Autodesk Inventor part; units mm, degrees
ref_plane "YZ Plane" through (0, 0, 0) normal (1, 0, 0) x (0, 1, 0)
ref_plane "XZ Plane" through (0, 0, 0) normal (0, 1, 0) x (-1, 0, 0)
ref_plane "XY Plane" through (0, 0, 0) normal (0, 0, 1) x (1, 0, 0)
sketch "Boceto1" plane through (0, 0, 0) normal (0, 1, 0) x (-1, 0, 0)
  circle A0 centre (0, 0) radius 34.5
  circle A1 centre (0, 0) radius 35
  dimension "d0" = 69
  dimension "d1" = 70
extrude "Extrusión1" add sketch "Boceto1" along normal blind 1 contours A0 | A1
sketch "Boceto2" plane through (0, 1, 0) normal (0, 1, 0) x (1, 0, 0)
  circle A0 centre (0, 0) radius 34.5
  circle A1 centre (0, 0) radius 35
  dimension "d4" = 69
  dimension "d5" = 70
extrude "Extrusión2" add sketch "Boceto2" along normal blind 25
sketch "Boceto3" plane through (0, 1, 0) normal (0, 1, 0) x (1, 0, 0)
  circle A0 centre (0, 0) radius 2.1
  circle A1 centre (0, 0) radius 1.75
  dimension "d8" = 4.2
  dimension "d9" = 3.5
extrude "Extrusión3" add sketch "Boceto3" along normal blind 3
sketch "Boceto4" plane through (0, 1, 0) normal (0, 1, 0) x (1, 0, 0)
  circle A0 centre (0, 0) radius 1.75
  dimension "d14" = 3.5
extrude "Extrusión4" cut sketch "Boceto4" against normal through all
properties part number "Molde"
Could you check a few things on this model? Use its own coordinates, in mm. A direction names the side the tool comes from. Coordinates: 2 decimals unless noted, no trailing zeros. Order: outer loops, then holes, each group sorted by start corner. A loop starts at its lowest first (then second) coordinate and runs counter-clockwise, first axis right, second up. Notation, with made-up numbers: M 41,-3.5 L 76,-3.5 A5 ccw 76,1.5 Z; hole C 89.25,42 d8. An arc over 180 degrees is marked long. Use a Markdown table: item, result. Add a question column.
Q1. I want a section at A-A on z = 0. List the corners of the cut face in (x, y) for me, then the cut area to 3 significant figures.
Q2. We'd pull the mould along Z, two halves only. Please class faces 1 (the cylindrical face through (32.907, 13.325, 10.363)), 2 (the flat face through (26, 26, 23)): pulls with the +Z half, pulls with the -Z half, needs draft (parallel to the pull), parting line crosses it, or undercut.
Q3. If I drill on L1, parallel to Z at x = 0, y = 2.95; L2, parallel to X at y = 0.6, z = 0; L3, parallel to Z at x = 0, y = 15.25, over which ranges is the centre line in solid material (lowest first)?
Q4. I'm going to push flat-ended pins straight in: pin 1 (5 mm diameter, centred on y = 4, z = -25.5, fed in from +X); pin 2 (1 mm diameter, centred on y = 3.5, z = -19.5, fed in from -X); pin 3 (5 mm diameter, centred on x = 24, y = 7, fed in from +Z). Where does each tip first touch, or does it pass through?
Q5. Which directions (+Z, -Z, +X, -X, +Y, -Y) give clear straight access to the entire face, cutting with the end or side of a thin tool? Please do faces 3 (the flat face through (0, 1, -7)), 4 (the flat face through (0, 0, -7)).
Q6. I want a section at D-D on y = 17. List the corners of the cut face in (x, z) for me.
Q7. I want a section at C-C on y = 2.5. List the corners of the cut face in (x, z) for me, then the cut area to 3 significant figures.
Q8. I want a section at B-B on x = 0. List the corners of the cut face in (y, z) for me.
Checked values:
| question | item | result |
|---|---|---|
| 1 | outline | M -35,0 L -1.75,0 L -1.75,4 L -2.1,4 L -2.1,1 L -34.5,1 L -34.5,26 L -35,26 Z; M 1.75,0 L 35,0 L 35,26 L 34.5,26 L 34.5,1 L 2.1,1 L 2.1,4 L 1.75,4 Z |
| 1 | area | 93.6 mm² |
| 2 | face 1 | undercut |
| 2 | face 2 | needs draft |
| 3 | L1 | -35 to -34.5, -2.1 to -1.75, 1.75 to 2.1, 34.5 to 35 |
| 3 | L2 | -35 to -1.75, 1.75 to 35 |
| 3 | L3 | -35 to -34.5, 34.5 to 35 |
| 4 | pin 1 | x = 26.38 |
| 4 | pin 2 | x = -29.39 |
| 4 | pin 3 | z = 27.62 |
| 5 | face 3 | +Y |
| 5 | face 4 | +Z, -Z, +X, -X, -Y |
| 6 | outline | C 0,0 d70; hole C 0,0 d69 |
| 7 | outline | C 0,0 d70; C 0,0 d4.2; hole C 0,0 d69; hole C 0,0 d3.5 |
| 7 | area | 113 mm² |
| 8 | outline | M 0,-35 L 26,-35 L 26,-34.5 L 1,-34.5 L 1,-2.1 L 4,-2.1 L 4,-1.75 L 0,-1.75 Z; M 0,1.75 L 4,1.75 L 4,2.1 L 1,2.1 L 1,34.5 L 26,34.5 L 26,35 L 0,35 Z |
